Part print with two shaded views. Sizes in mm from the minimum x, y, z corner. Coordinates: 2 decimals unless noted, no trailing zeros. Write each loop counter-clockwise with the first axis right and the second up, starting at its lowest first coordinate (ties: lowest second). Pieces come first, ordered by that corner, then holes. Notation, with made-up numbers: (-19, 89) - (-2, 89) arc R30 cw to (-2, 124) - close; hole circle Ø6 at (-13, 19). An arc over 180 degrees is marked (long way). Answer in a Markdown table with one row per item. Add a question column.
Q1. Pin check, flat tip, straight feed: pin 1 (12.5 mm diameter, centred on y = 15.5, z = 13, fed in from +X). Stop position of the tip, or through.
Q2. Band-saw the part on B-B (y = 42). List the corners of the cut face in (x, z).
Q3. Band-saw the part on C-C (x = 75.5). List the corners of the cut face in (y, z) (1 decimal).
Q4. Drill centre lines: line 1 along Y through (x, z) = (12.5, 7); line 2 along Y through (x, z) = (80.5, 2.5) (1 decimal). Where is each one in solid material? Low to high. Write a range as from..to.
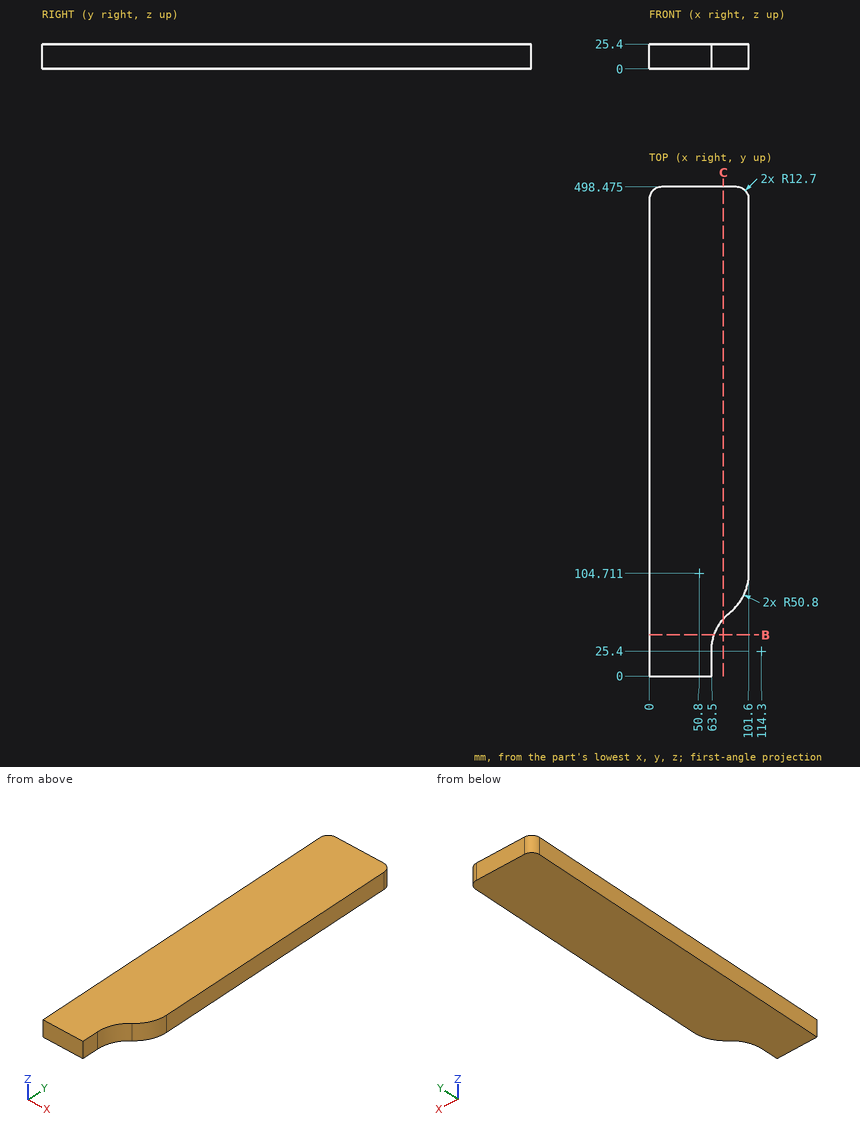
Checked values:
| question | item | result |
|---|---|---|
| 1 | pin 1 | stops at x = 63.5 |
| 2 | outline | (0, 0) - (66.29, 0) - (66.29, 25.4) - (0, 25.4) - close |
| 3 | outline | (58.2, 0) - (498.5, 0) - (498.5, 25.4) - (58.2, 25.4) - close |
| 4 | line 1 | y = 0..498.47 |
| 4 | line 2 | y = 63.3..498.5 |
